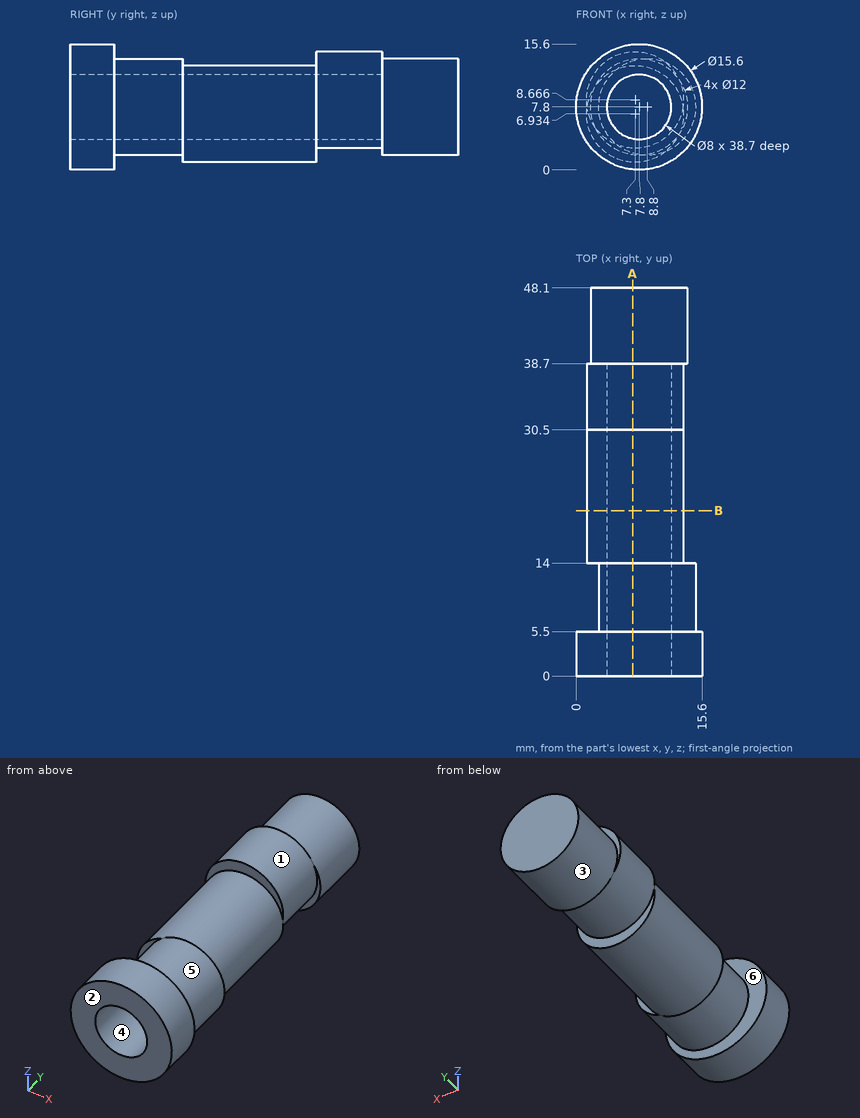
Can you work these out from the drawing? Everything is in mm from the part's minimum corner. A direction names the side the tool comes from. Round coordinates to 2 decimals unless told otherwise and drop trailing zeros. Loops run counter-clockwise (first coordinate to the right, second up) from the corner with the lowest first, then second, coordinate; pieces in that order, holes last. Notation, with made-up numbers: (-3.5, 53) - (29.5, 53) arc R9 cw to (29.5, 66) - close; hole circle Ø6 at (50, -39). An arc over 180 degrees is marked (long way). Write item = value, one per line. Start each with the question number.
(1) If we mould it in two halves opening along Z, with no side actions, what happens to the marked faces 4, 5 and 6? For each: released by +Z, released by -Z, zero draft, split by the parting line, or undercut.
(2) If I drill on probe 1 along Y at (x, z) = (3.75, 11.25); probe 2 along Y at (x, z) = (7, 1.5); probe 3 along X at (y, z) = (10.5, 7.8), over which ranges is the centre line in solid material (lowest first)? Write a range as [from, to].
(3) For the marked faces 1, 2 and 3, which set-ups out of +Z, -Z, +X, -X, +Y, -Y let a thin tool reach every point of the face, with its end or its side?
(4) If we section it at A-A (x = 7): Please give me the cut outline in (y, z), and give its area (3 significant figures).
(5) For P1, Ø1, axis at x = 12, y = 23.5, coming from the -Z side; P2, Ø8, axis at x = 2.5, y = 41.5, coming from the -Z side; P3, Ø4, axis at x = 8.5, y = 15, coming from the -Z side, each with a flat end and sliding along its axis, tell me the tip position at first contact or that it passes through.
(6) If we section it at B-B (y = 20.5): Please give me the cut outline in (x, z).
Ans:
q1.face_4 = undercut
q1.face_5 = split by the parting line
q1.face_6 = zero draft
q2.probe_1 = [0, 5.5], [14, 48.1]
q2.probe_2 = [0, 5.5], [14, 30.5]
q2.probe_3 = [2.8, 3.8], [11.8, 14.8]
q3.face_1 = none
q3.face_2 = +Z, -Z, +X, -X, -Y
q3.face_3 = +Y
q4.outline = (0, 0.04) - (5.5, 0.04) - (5.5, 2.08) - (14, 2.08) - (14, 0.94) - (30.5, 0.94) - (30.5, 2.67) - (38.7, 2.67) - (38.7, 1.85) - (48.1, 1.85) - (48.1, 13.75) - (38.7, 13.75) - (38.7, 14.66) - (30.5, 14.66) - (30.5, 12.93) - (14, 12.93) - (14, 13.52) - (5.5, 13.52) - (5.5, 15.56) - (0, 15.56) - (0, 11.72) - (38.7, 11.72) - (38.7, 3.88) - (0, 3.88) - close
q4.area = 287 mm²
q5.P1 = 2.65
q5.P2 = 1.94
q5.P3 = 0.93
q6.outline = circle Ø12 at (7.3, 6.93); hole circle Ø8 at (7.8, 7.8)
